Check sheet for the modelled part. Datum: model origin and axes. Units: mm. A direction names the side the tool comes from. Coordinates: 2 decimals unless noted, no trailing zeros. Order: outer loops, then holes, each group sorted by start corner. A loop starts at its lowest first (then second) coordinate and runs counter-clockwise, first axis right, second up.
from build123d import *

# Parameters (mm, degrees)
BOSS_EXTRUDE1_DEPTH       = 6.35
F_6_CLEARANCE_HOLE1_D     = 3.7973
F_6_CLEARANCE_HOLE1_DEPTH = 6.733175986
F_6_CLEARANCE_HOLE1_TIP   = 1.140824014
FILLET1_R                 = 0.508


with BuildPart() as part:
    # Sketch1 → Boss-Extrude1 (new body)
    with BuildSketch(Plane(origin=(0, 0, 0), x_dir=(1, 0, 0), z_dir=(0, 1, 0))):
        Polygon((11.567845271, -11.620817646), (16.838662917, -6.35), (16.838662917, 12.7), (10.488662917, 12.7), (10.488662917, -6.35), (6.297027625, -6.35), align=None)
    extrude(amount=BOSS_EXTRUDE1_DEPTH)

    # #6 Clearance Hole1
    with Locations(Plane.ZY.offset(-10.488662917)):
        with Locations((-8.89, 3.175), (2.54, 3.175)):
            Hole(F_6_CLEARANCE_HOLE1_D / 2, depth=F_6_CLEARANCE_HOLE1_DEPTH)
            with Locations((0, 0, -(F_6_CLEARANCE_HOLE1_DEPTH + F_6_CLEARANCE_HOLE1_TIP / 2))):  # 118° drill point
                Cone(0, F_6_CLEARANCE_HOLE1_D / 2, F_6_CLEARANCE_HOLE1_TIP, mode=Mode.SUBTRACT)

    # Fillet1
    fillet1_edges = [part.edges().sort_by_distance(p)[0] for p in [
        (6.297027625, 3.175, 6.35),
        (10.488662917, 3.175, 6.35),
        (16.838662917, 3.175, 6.35),
        (11.567845271, 3.175, 11.620817646),
    ]]
    fillet(fillet1_edges, radius=FILLET1_R)


solid = part.part
(1) Tool access check on faces 4 (the flat face through (16.839, 3, -3)), 5 (the flat face through (10.489, 3, -4)). Record the directions out of +Z, -Z, +X, -X, +Y, -Y that give a thin tool (end or side, any length) a straight path to the whole face; none if there is none.
Filled in:
face 4: +Z, -Z, +X, +Y, -Y
face 5: -Z, -X, +Y, -Y
(2) Cross-section at A-A (z = -8.89). Enter the section's corners in (x, y).
Filled in:
outline: (10.49, 0) - (16.84, 0) - (16.84, 1.28) - (10.49, 1.28) - close; (10.49, 5.07) - (16.84, 5.07) - (16.84, 6.35) - (10.49, 6.35) - close
(3) Cross-section at C-C (z = 3.5). Enter the section's corners in (x, y).
Filled in:
outline: (10.49, 0) - (16.84, 0) - (16.84, 1.54) - (10.49, 1.54) - close; (10.49, 4.81) - (16.84, 4.81) - (16.84, 6.35) - (10.49, 6.35) - close
(4) Go/stop test with flat-tipped pins: P1, Ø2, axis at x = 8.5, y = 2, coming from the -Z side; P2, Ø1.5, axis at y = 1, z = 8, coming from the -X side; P3, Ø1.9, axis at y = 3, z = -1.5, coming from the -X side. Record where each tip stops, or that it passes through.
Filled in:
P1: stops at z = 6.35
P2: stops at x = 7.2
P3: stops at x = 10.49
(5) Cross-section at D-D (y = 3.75). Enter the section's corners in (x, z), and give its area (3 significant figures).
Filled in:
outline: (7.16, 7.22) arc R0.51 ccw to (7.52, 6.35) - (9.98, 6.35) arc R0.51 cw to (10.49, 5.84) - (10.49, 4.35) - (16.84, 4.35) - (16.84, 6.14) arc R0.51 ccw to (16.69, 6.5) - (11.93, 11.26) arc R0.51 ccw to (11.21, 11.26) - close; (10.49, -12.7) - (16.84, -12.7) - (16.84, -10.7) - (10.49, -10.7) - close; (10.49, -7.08) - (16.84, -7.08) - (16.84, 0.73) - (10.49, 0.73) - close
area: 102 mm2
(6) Cross-section at B-B (y = 2.5). Enter the section's corners in (x, z), and give its area (3 significant figures).
Filled in:
outline: (7.16, 7.22) arc R0.51 ccw to (7.52, 6.35) - (9.98, 6.35) arc R0.51 cw to (10.49, 5.84) - (10.49, 4.31) - (16.84, 4.31) - (16.84, 6.14) arc R0.51 ccw to (16.69, 6.5) - (11.93, 11.26) arc R0.51 ccw to (11.21, 11.26) - close; (10.49, -12.7) - (16.84, -12.7) - (16.84, -10.66) - (10.49, -10.66) - close; (10.49, -7.12) - (16.84, -7.12) - (16.84, 0.77) - (10.49, 0.77) - close
area: 103 mm2
(7) Thickness scan on probe 1 along Y at (x, z) = (15.5, 2.54); probe 2 along Z at (x, y) = (12.75, 2.5); probe 3 along Z at (x, y) = (12, 3.75). Record the ranges inside material, lowest first.
Filled in:
probe 1: y = 0 to 1.28, 5.07 to 6.35
probe 2: z = -12.7 to -10.66, -7.12 to 0.77, 4.31 to 10.44
probe 3: z = -12.7 to -10.7, -7.08 to 0.73, 4.35 to 11.19
(8) Release check for a two-part mould opening along Y. For faces 1 (the cylindrical face through (14, 3, -7)), 2 (the flat face through (13, 6.35, -1)), 3 (the flat face through (9.158, 3.131, 9.211)) record: +Y half, -Y half, draft (parallel to the pull), parting line (faces both ways), or undercut.
Filled in:
face 1: undercut
face 2: +Y half
face 3: draft
